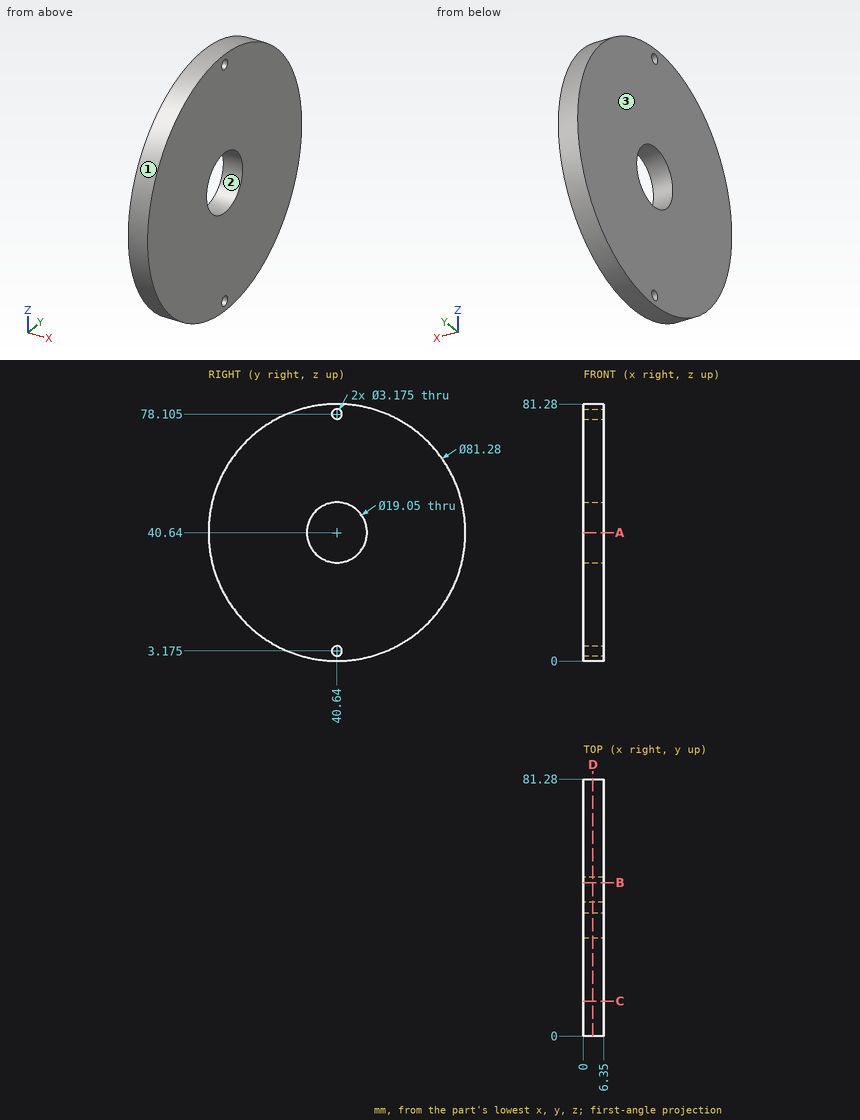
Input: dimensioned drawing with shaded views. Units: mm. Origin: part minimum x, y, z. Coordinates: 2 decimals unless noted, no trailing zeros. Loops run counter-clockwise (first coordinate to the right, second up) from the corner with the lowest first, then second, coordinate; pieces in that order, holes last. Notation, with made-up numbers: M 43,21.25 L 89,21.25 A12 ccw 89,38.25 Z; hole C 79.25,29.5 d8. An arc over 180 degrees is marked long. Use a Markdown table: item, result. Add a question column.
1) Pin query (flat end, axial travel): P1, Ø3, axis at y = 40.64, z = 78.105, coming from the -X side; P2, Ø3, axis at x = 3, z = 27, coming from the +Y side; P3, Ø3, axis at x = 5, y = 40, coming from the -Z side; P4, Ø3, axis at x = 4.5, z = 26, coming from the -Y side. Return the tip coordinate at first contact, or that it passes through.
2) Section B-B, the plane y = 48.5. Return the cut outline in (x, z), plus the area to 3 significant figures.
3) Line query: L1, parallel to Z at x = 4, y = 40.64 (1 decimal); L2, parallel to Y at x = 6, z = 35; L3, parallel to Y at x = 4, z = 36. Output: solid intervals per line, ascending. Write a range as from..to.
4) Section D-D, the plane x = 3. Give the number of separate pieces and of enclosed holes in the cut face, plus the area to 3 significant figures.
5) Section C-C, the plane y = 11. Return the cut outline in (x, z).
6) Section A-A, the plane z = 40.64. Return the cut outline in (x, y) (3 decimals).
7) Draft query along Z for the marked faces 1, 2 and 3. Return one class per face: +Z half, -Z half, draft (parallel to the pull), parting line (faces both ways), or undercut.
Answer below:
| question | item | result |
|---|---|---|
| 1 | P1 | through |
| 1 | P2 | y = 79.42 |
| 1 | P3 | z = 0 |
| 1 | P4 | y = 2.18 |
| 2 | outline | M 0,0.77 L 6.35,0.77 L 6.35,35.26 L 0,35.26 Z; M 0,46.02 L 6.35,46.02 L 6.35,80.51 L 0,80.51 Z |
| 2 | area | 438 mm2 |
| 3 | L1 | 0..1.6, 4.8..31.1, 50.2..76.5, 79.7..81.3 |
| 3 | L2 | 0.39..32.96, 48.32..80.89 |
| 3 | L3 | 0.27..32.32, 48.96..81.01 |
| 4 | separate pieces | 1 |
| 4 | enclosed holes | 3 |
| 4 | area | 4,890 mm2 |
| 5 | outline | M 0,12.84 L 6.35,12.84 L 6.35,68.44 L 0,68.44 Z |
| 6 | outline | M 0,0 L 6.35,0 L 6.35,31.115 L 0,31.115 Z; M 0,50.165 L 6.35,50.165 L 6.35,81.28 L 0,81.28 Z |
| 7 | face 1 | parting line |
| 7 | face 2 | undercut |
| 7 | face 3 | draft |
